Input: part model. Units: mm. Frame: model coordinates. Coordinates: 2 decimals unless noted, no trailing zeros. Order: outer loops, then holes, each group sorted by start corner. A loop starts at its lowest first (then second) coordinate and runs counter-clockwise, first axis right, second up. Notation, with made-up numbers: M 4,44 L 29,44 A27 cw 29,72 Z; hole C 2.5,26.5 d4. An arc over 180 degrees is marked long. One line per item, written item: value.
```python
from build123d import *

# Parameters (mm, degrees)
SKETCH1_W           = 1771.65
SKETCH1_H           = 88.9
BOSS_EXTRUDE1_DEPTH = 38.1
CUT_EXTRUDE1_DEPTH  = 89.9
SKETCH3_W           = 84.1375
SKETCH3_H           = 50.8
CUT_EXTRUDE2_DEPTH  = 39.1


with BuildPart() as part:
    # Sketch1 → Boss-Extrude1 (new body)
    with BuildSketch(Plane(origin=(0, 0, 0), x_dir=(1, 0, 0), z_dir=(0, 1, 0))):
        with Locations((885.825, 44.45)):
            Rectangle(SKETCH1_W, SKETCH1_H)
    extrude(amount=BOSS_EXTRUDE1_DEPTH)

    # Sketch2 → Cut-Extrude1 (cut, through all)
    with BuildSketch(Plane.XY):
        Polygon((0, 0), (38.1, 38.1), (0, 38.1), align=None)
        Polygon((1771.65, 0), (1771.65, 38.1), (1733.55, 38.1), align=None)
    extrude(amount=-CUT_EXTRUDE1_DEPTH, mode=Mode.SUBTRACT)

    # Sketch3 → Cut-Extrude2 (cut, through all)
    with BuildSketch(Plane.XZ):
        with Locations((516.73125, -25.4)):
            Rectangle(SKETCH3_W, SKETCH3_H)
    extrude(amount=-CUT_EXTRUDE2_DEPTH, mode=Mode.SUBTRACT)


solid = part.part
```
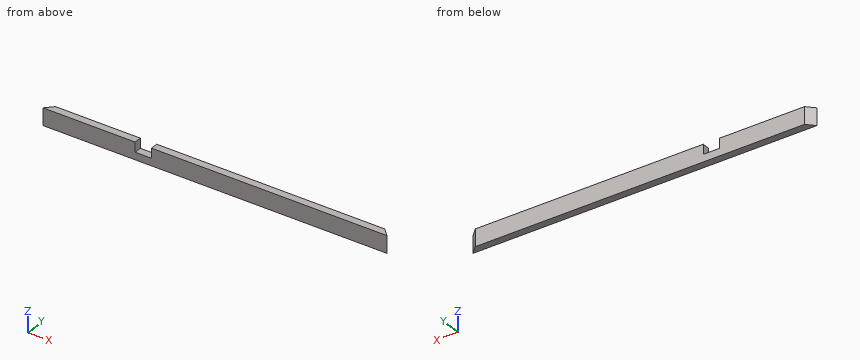
(1) Cut plane B-B on y = 7. Output: boundary loops of the cut face in (x, z), plus the area to 3 significant figures.
Data:
outline: M 7,-88.9 L 1764.65,-88.9 L 1764.65,0 L 558.8,0 L 558.8,-50.8 L 474.66,-50.8 L 474.66,0 L 7,0 Z
area: 152,000 mm2
(2) Ray query, line 1 (X direction, y = 35, z = -41); line 2 (X direction, y = 22, z = -24); line 3 (Z direction, x = 546.5, y = 28.5). Return the intervals inside material, ascending. Write a range as from..to.
Data:
line 1: x = 35..474.66, 558.8..1736.65
line 2: x = 22..474.66, 558.8..1749.65
line 3: z = -88.9..-50.8
(3) Cut plane A-A on z = -14. Output: boundary loops of the cut face in (x, y), plus the area to 3 significant figures.
Data:
outline: M 0,0 L 474.66,0 L 474.66,38.1 L 38.1,38.1 Z; M 558.8,0 L 1771.65,0 L 1733.55,38.1 L 558.8,38.1 Z
area: 62,800 mm2
(4) First-contact query: pin 1 (11.5 mm diameter, centred on y = 13, z = -35, fed in from +X); pin 2 (12 mm diameter, centred on y = 21.5, z = -26, fed in from -X); pin 3 (6 mm diameter, centred on y = 9, z = -62.5, fed in from -X). Flat tips, straight axial feed; report the tip coordinate or a pass-through.
Data:
pin 1: stops at x = 1764.4
pin 2: stops at x = 15.5
pin 3: stops at x = 6
